Design review of the part built by this model. Coordinates are the model's own, in mm. Round coordinates to 2 decimals unless told otherwise and drop trailing zeros. Loops run counter-clockwise (first coordinate to the right, second up) from the corner with the lowest first, then second, coordinate; pieces in that order, holes last. Notation, with made-up numbers: M -11,-8 L 40,-8 A22 ccw 40,18 Z; hole C 34.25,5.5 d8. An arc over 180 degrees is marked long. One line per item, written item: value. Start each with the question number.
Item 1: We need section D-D (z = -120). Write out the cut boundary in (x, y).
Item 2: For line 1 along X through (y, z) = (1.8, 120); line 2 along Z through (x, y) = (0, 2.25); line 3 along X through (y, z) = (1.4, 0), list the stretches that pass through material, from the lowest coordinate up.
Item 3: We need section A-A (y = 1.4). Write out the cut boundary in (x, z).
Item 4: Mouldability with a two-part tool opening along Z and no side actions: class faces 1 (the cylindrical face through (33.759, 1.479, -122.974)), 2 (the cylindrical face through (-28, 1, 21)), 3 (the flat face through (-21, 3, -31)) as released by +Z, released by -Z, zero draft, split by the parting line, or undercut.
Item 5: We need section C-C (x = 0). Write out the cut boundary in (y, z).
Item 6: We need section B-B (z = 0). Write out the cut boundary in (x, y).
from build123d import *

# Parameters (mm, degrees)
SKETCH1_W           = 90
SKETCH1_H           = 260
SKETCH1_R           = 35
SKETCH1_R_2         = 3
BOSS_EXTRUDE1_DEPTH = 3
FILLET1_R           = 3


with BuildPart() as part:
    # Sketch1 → Boss-Extrude1 (new body)
    with BuildSketch(Plane(origin=(0, 0, 0), x_dir=(1, 0, 0), z_dir=(0, 1, 0))):
        Rectangle(SKETCH1_W, SKETCH1_H)
        Circle(SKETCH1_R, mode=Mode.SUBTRACT)
        with Locations((-34.15, 120)):
            Circle(SKETCH1_R_2, mode=Mode.SUBTRACT)
        with Locations((34.15, 120)):
            Circle(SKETCH1_R_2, mode=Mode.SUBTRACT)
        with Locations((34.15, -120)):
            Circle(SKETCH1_R_2, mode=Mode.SUBTRACT)
        with Locations((-34.15, -120)):
            Circle(SKETCH1_R_2, mode=Mode.SUBTRACT)
    extrude(amount=BOSS_EXTRUDE1_DEPTH)

    # Fillet1
    fillet1_edges = [part.edges().sort_by_distance(p)[0] for p in [
        (45, 1.5, 130),
        (-45, 1.5, 130),
        (-45, 1.5, -130),
        (45, 1.5, -130),
    ]]
    fillet(fillet1_edges, radius=FILLET1_R)


solid = part.part
A:
1. outline: M -45,0 L -37.15,0 L -37.15,3 L -45,3 Z; M -31.15,0 L 31.15,0 L 31.15,3 L -31.15,3 Z; M 37.15,0 L 45,0 L 45,3 L 37.15,3 Z
2. line 1: -45 to -37.15, -31.15 to 31.15, 37.15 to 45
2. line 2: -130 to -35, 35 to 130
2. line 3: -45 to -35, 35 to 45
3. outline: M -45,-127 A3 ccw -42,-130 L 42,-130 A3 ccw 45,-127 L 45,127 A3 ccw 42,130 L -42,130 A3 ccw -45,127 Z; hole C -34.15,-120 d6; hole C -34.15,120 d6; hole C 0,0 d70; hole C 34.15,-120 d6; hole C 34.15,120 d6
4. face 1: undercut
4. face 2: undercut
4. face 3: zero draft
5. outline: M 0,-130 L 3,-130 L 3,-35 L 0,-35 Z; M 0,35 L 3,35 L 3,130 L 0,130 Z
6. outline: M -45,0 L -35,0 L -35,3 L -45,3 Z; M 35,0 L 45,0 L 45,3 L 35,3 Z
